Geometry check sheet. Reference: the model listing, model coordinates, mm. A direction names the side the tool comes from. Round coordinates to 2 decimals unless told otherwise and drop trailing zeros. Order: outer loops, then holes, each group sorted by start corner. A loop starts at its lowest first (then second) coordinate and runs counter-clockwise, first axis right, second up. Notation, with made-up numbers: (87, 44.5) - (101, 44.5) arc R21 cw to (101, 67.5) - close; hole circle Ø5 at (-1.75, -12). An arc over 180 degrees is marked (long way). Use a Markdown table: item, result. Add a question column.
(1) Mould release check, pull along X, two halves, no side actions. Record for faces 1 (the face through (-17.47, -40.28, 1.61)), 2 (the face through (-16, -41, 0)), 3 (the face through (-27.54, -41.19, -13.11)): released by +X, released by -X, zero draft, split by the parting line, or undercut.
(2) Gauge pin test, flat ends, axial feed: P1, Ø1.1, axis at x = -1.5, y = -30, coming from the +Z side; P2, Ø8, axis at x = -21, z = 5.5, coming from the +Y side; P3, Ø5, axis at x = -27, y = 0.5, coming from the -Z side; P4, Ø3.5, axis at x = -20, z = 0, coming from the -Y side. Record the tip position at first contact, or that the pin passes through.
(3) Section check A-A on x = -5.5. Record the boundary of the cut face in (y, z), then the cut area to 3 significant figures.
(4) Section check D-D on z = 1. Give the number of separate pieces and of enclosed holes in the cut face, then the cut area to 3 significant figures.
(5) Thickness scan on line 1 along Y through (x, z) = (-17, 2); line 2 along Y through (x, z) = (-27, 12); line 3 along Z through (x, y) = (-26.5, -30.2). Record the ranges inside material, lowest first. Write a range as [from, to].
(6) Section check B-B on z = 12.5. Record the boundary of the cut face in (x, y), then the cut area to 3 significant figures.
(7) Section check C-C on y = -12.5. Record the boundary of the cut face in (x, z).
(8) Access from +Z, -Z, +X, -X, +Y, -Y to the whole of each face (thin tool, end or side, straight path). Record for faces 4 (the face through (-8, 3, -5)), 5 (the face through (-27, -4, -13)), 6 (the face through (-19, 1, 5)).
```python
from build123d import *

# Parameters (mm, degrees)
CROQUIS1_R              = 3
CROQUIS1_R_2            = 3.1
SALIENTE_EXTRUIR1_DEPTH = 6
CROQUIS2_W              = 10
CROQUIS2_H              = 3
SALIENTE_EXTRUIR2_DEPTH = 14.2
SALIENTE_EXTRUIR3_START = 24.5
CROQUIS3_R              = 3.1
SALIENTE_EXTRUIR3_DEPTH = 24.5
CROQUIS6_R              = 8
CORTAR_EXTRUIR1_DEPTH   = 18
REDONDEO1_R             = 5
CROQUIS7_W              = 17.859034053
CROQUIS7_H              = 1
CORTAR_EXTRUIR2_DEPTH   = 1
CROQUIS8_W              = 13
CROQUIS8_H              = 6
SALIENTE_EXTRUIR4_DEPTH = 20
CROQUIS9_W              = 5
CROQUIS9_H              = 13
SALIENTE_EXTRUIR5_DEPTH = 20.2
CROQUIS10_W             = 3
CROQUIS10_H             = 14.2
CORTAR_EXTRUIR3_DEPTH   = 20
SALIENTE_EXTRUIR6_DEPTH = 5
SALIENTE_EXTRUIR7_DEPTH = 6
REDONDEO2_R             = 4
CROQUIS13_W             = 15
CROQUIS13_H             = 24.5
CORTAR_EXTRUIR4_DEPTH   = 11
REDONDEO3_R             = 4
REDONDEO4_R             = 5
REDONDEO9_SIZE          = 10
CROQUIS15_W             = 23.51054635
CROQUIS15_H             = 8.430737454
CORTAR_EXTRUIR6_DEPTH   = 12.311914061
REDONDEO10_R            = 5
CROQUIS16_W             = 33
CROQUIS16_H             = 33
SALIENTE_EXTRUIR8_DEPTH = 5
CROQUIS18_R             = 1.5
CORTAR_EXTRUIR7_DEPTH   = 10
CROQUIS19_R             = 8
CORTAR_EXTRUIR8_DEPTH   = 10
REDONDEO13_R            = 5
REDONDEO14_R            = 5
REDONDEO15_R            = 5
REDONDEO17_SIZE         = 3
CROQUIS20_W             = 26.447439695
CROQUIS20_H             = 7.153283898
CORTAR_EXTRUIR9_DEPTH   = 8
REDONDEO18_DEPTH        = 6
REDONDEO19_SIZE         = 4
REDONDEO20_SIZE         = 5
CROQUIS21_W             = 10
CROQUIS21_H             = 4.320063387
SALIENTE_EXTRUIR9_DEPTH = 9
CROQUIS14_R             = 3
CORTAR_EXTRUIR5_DEPTH   = 59


with BuildPart() as part:
    # Croquis1 → Saliente-Extruir1 (new body)
    with BuildSketch(Plane(origin=(0, 0, 0), x_dir=(1, 0, 0), z_dir=(0, 1, 0))):
        with BuildLine():
            Line((-5, 20), (-5, 0))
            ThreePointArc((-5, 0), (0, -5), (5, 0))
            Line((5, 0), (5, 20))
            ThreePointArc((5, 20), (0, 25), (-5, 20))
        make_face()
        with Locations(Location((0, 20, 0), (0, 0, 270))):
            Circle(CROQUIS1_R, mode=Mode.SUBTRACT)
        with Locations(Location((0, 0, 0), (0, 0, 270))):
            Circle(CROQUIS1_R_2, mode=Mode.SUBTRACT)
    extrude(amount=SALIENTE_EXTRUIR1_DEPTH)

    # Croquis2 → Saliente-Extruir2 (add)
    with BuildSketch(Plane.XZ):
        with Locations((0, -14.5)):
            Rectangle(CROQUIS2_W, CROQUIS2_H)
    extrude(amount=SALIENTE_EXTRUIR2_DEPTH)

    # Croquis3 → Saliente-Extruir3 (add)
    with BuildSketch(Plane.XZ.offset(14.2).offset(SALIENTE_EXTRUIR3_START)):
        with BuildLine():
            Line((-5, -5), (-5, -16))
            Line((-5, -16), (5, -16))
            Line((5, -16), (5, 0))
            ThreePointArc((5, 0), (3.535533906, 3.535533906), (0, 5))
            Line((0, 5), (-30, 5))
            Line((-30, 5), (-30, -5))
            Line((-30, -5), (-5, -5))
        make_face()
        with Locations(Location((0, 0, 0), (0, 0, 90))):
            Circle(CROQUIS3_R, mode=Mode.SUBTRACT)
    extrude(amount=-SALIENTE_EXTRUIR3_DEPTH)

    # Croquis6 → Cortar-Extruir1 (cut)
    with BuildSketch(Plane.XY.offset(5)):
        with Locations((-20, -30.2)):
            Circle(CROQUIS6_R)
    extrude(amount=-CORTAR_EXTRUIR1_DEPTH, mode=Mode.SUBTRACT)

    # Redondeo1
    redondeo1_edges = [part.edges().sort_by_distance(p)[0] for p in [
        (-5, -26.45, -5),
    ]]
    fillet(redondeo1_edges, radius=REDONDEO1_R)

    # Croquis7 → Cortar-Extruir2 (cut)
    with BuildSketch(Plane.XY.offset(5)):
        with Locations((-3.905990917, -30.2)):
            Rectangle(CROQUIS7_W, CROQUIS7_H)
    extrude(amount=-CORTAR_EXTRUIR2_DEPTH, mode=Mode.SUBTRACT)

    # Croquis8 → Saliente-Extruir4 (add)
    with BuildSketch(Plane.ZY.offset(5)):
        with Locations((-6.5, 3)):
            Rectangle(CROQUIS8_W, CROQUIS8_H)
    extrude(amount=SALIENTE_EXTRUIR4_DEPTH)

    # Croquis9 → Saliente-Extruir5 (add)
    with BuildSketch(Plane(origin=(0, 6, 0), x_dir=(1, 0, 0), z_dir=(0, 1, 0))):
        with Locations((-27.5, 6.5)):
            Rectangle(CROQUIS9_W, CROQUIS9_H)
    extrude(amount=-SALIENTE_EXTRUIR5_DEPTH)

    # Croquis10 → Cortar-Extruir3 (cut)
    with BuildSketch(Plane.ZY.offset(5)):
        with Locations((-14.5, -7.1)):
            Rectangle(CROQUIS10_W, CROQUIS10_H)
    extrude(amount=-CORTAR_EXTRUIR3_DEPTH, mode=Mode.SUBTRACT)

    # Croquis11 → Saliente-Extruir6 (add)
    with BuildSketch(Plane.XY):
        Polygon((-5, 0), (-5, 6), (-30, 6), (-30, -14.2), (-25, -14.2), (-25, 0), align=None)
    extrude(amount=SALIENTE_EXTRUIR6_DEPTH)

    # Croquis12 → Saliente-Extruir7 (add)
    with BuildSketch(Plane(origin=(0, 6, 0), x_dir=(1, 0, 0), z_dir=(0, 1, 0))):
        Polygon((-5, -5), (0, -5), (-4.695965468, 0.35178881), (-6.407055534, -0.228241721), align=None)
    extrude(amount=-SALIENTE_EXTRUIR7_DEPTH)

    # Redondeo2
    # the kernel refuses this fillet: 4 mm, written as the material it adds along each edge
    with BuildSketch(Plane(origin=(-30, -14.2, -5), x_dir=(0, 0, -1), z_dir=(1, 0, 0))) as redondeo2_piece_1:
        with BuildLine():
            CenterArc((REDONDEO2_R, -REDONDEO2_R), REDONDEO2_R, 90, 90)
            Line((0, -REDONDEO2_R), (0, 0))
            Line((0, 0), (REDONDEO2_R, 0))
        make_face()
    extrude(amount=5)

    # Croquis13 → Cortar-Extruir4 (cut)
    with BuildSketch(Plane(origin=(0, 0, -16), x_dir=(-1, 0, 0), z_dir=(0, 0, -1))):
        with Locations((2.5, -26.45)):
            Rectangle(CROQUIS13_W, CROQUIS13_H)
    extrude(amount=-CORTAR_EXTRUIR4_DEPTH, mode=Mode.SUBTRACT)

    # Redondeo3
    redondeo3_edges = [part.edges().sort_by_distance(p)[0] for p in [
        (-5, 3, -13),
    ]]
    fillet(redondeo3_edges, radius=REDONDEO3_R)

    # Redondeo4
    redondeo4_edges = [part.edges().sort_by_distance(p)[0] for p in [
        (5, -26.45, -5),
    ]]
    fillet(redondeo4_edges, radius=REDONDEO4_R - 0.0001)  # a hair under: the kernel refuses the full size

    # Redondeo9
    # a fillet whose section is not a circle: 10 mm, written as the material it takes off along each edge
    with BuildSketch(Plane(origin=(-30, 6, 30), x_dir=(0, -1, 0), z_dir=(0, 0, -1))) as redondeo9_piece_1:
        with BuildLine():
            Bezier((REDONDEO9_SIZE, 0), (0, 0), (0, -REDONDEO9_SIZE), weights=[1, 1, 1])
            Line((0, -REDONDEO9_SIZE), (0, 0))
            Line((0, 0), (REDONDEO9_SIZE, 0))
        make_face()
    extrude(amount=68, mode=Mode.SUBTRACT)

    # Croquis15 → Cortar-Extruir6 (cut)
    with BuildSketch(Plane.XY.offset(-25.311914061)):
        with Locations((-4.843890072, 4.215368727)):
            Rectangle(CROQUIS15_W, CROQUIS15_H)
    extrude(amount=CORTAR_EXTRUIR6_DEPTH, mode=Mode.SUBTRACT)

    # Redondeo10
    redondeo10_edges = [part.edges().sort_by_distance(p)[0] for p in [
        (5, 3, -13),
    ]]
    fillet(redondeo10_edges, radius=REDONDEO10_R)

    # Croquis16 → Saliente-Extruir8 (add)
    with BuildSketch(Plane.ZY.offset(30)):
        with Locations((0, -30.2)):
            Rectangle(CROQUIS16_W, CROQUIS16_H)
    extrude(amount=-SALIENTE_EXTRUIR8_DEPTH)

    # Croquis18 → Cortar-Extruir7 (cut)
    with BuildSketch(Plane.ZY.offset(30)):
        with Locations((12, -42.2)):
            Circle(CROQUIS18_R)
        with Locations((-12, -42.2)):
            Circle(CROQUIS18_R)
        with Locations((-12, -18.2)):
            Circle(CROQUIS18_R)
        with Locations((12, -18.2)):
            Circle(CROQUIS18_R)
    extrude(amount=-CORTAR_EXTRUIR7_DEPTH, mode=Mode.SUBTRACT)

    # Croquis19 → Cortar-Extruir8 (cut)
    with BuildSketch(Plane.ZY.offset(30)):
        with Locations((0, -30.2)):
            Circle(CROQUIS19_R)
    extrude(amount=-CORTAR_EXTRUIR8_DEPTH, mode=Mode.SUBTRACT)

    # Redondeo13
    redondeo13_edges = [part.edges().sort_by_distance(p)[0] for p in [
        (-27.5, -13.7, 16.5),
    ]]
    fillet(redondeo13_edges, radius=REDONDEO13_R)

    # Redondeo14
    redondeo14_edges = [part.edges().sort_by_distance(p)[0] for p in [
        (-27.5, -46.7, 16.5),
    ]]
    fillet(redondeo14_edges, radius=REDONDEO14_R)

    # Redondeo15
    redondeo15_edges = [part.edges().sort_by_distance(p)[0] for p in [
        (-27.5, -46.7, -16.5),
    ]]
    fillet(redondeo15_edges, radius=REDONDEO15_R)

    # Redondeo17
    # a fillet whose section is not a circle: 3 mm, written as the material it takes off along each edge
    with BuildSketch(Plane(origin=(-37.5, -13.7, -16.5), x_dir=(0, -1, 0), z_dir=(1, 0, 0))) as redondeo17_piece_1:
        with BuildLine():
            Bezier((REDONDEO17_SIZE, 0), (0, 0), (0, -REDONDEO17_SIZE), weights=[1, 1, 1])
            Line((0, -REDONDEO17_SIZE), (0, 0))
            Line((0, 0), (REDONDEO17_SIZE, 0))
        make_face()
    extrude(amount=20, mode=Mode.SUBTRACT)

    # Croquis20 → Cortar-Extruir9 (cut)
    with BuildSketch(Plane(origin=(0, 0, -13), x_dir=(-1, 0, 0), z_dir=(0, 0, -1))):
        with Locations((6.776280153, 2.423358051)):
            Rectangle(CROQUIS20_W, CROQUIS20_H)
    extrude(amount=-CORTAR_EXTRUIR9_DEPTH, mode=Mode.SUBTRACT)

    # Redondeo18: read off the stored shape, not the designer's step
    # Redondeo18 outline → Redondeo18 (add)
    with BuildSketch(Plane(origin=(0, 0, 0), x_dir=(1, 0, 0), z_dir=(0, 1, 0))):
        with BuildLine():
            Line((-20, 5), (-16, 5))
            add(Edge.make_bspline(
                [(-16, 5), (-20, 5), (-20, 9)],
                knots=[0, 0, 0, 1, 1, 1], degree=2))
            Line((-20, 9), (-20, 5))
        make_face()
    extrude(amount=REDONDEO18_DEPTH)

    # Redondeo19
    # a fillet whose section is not a circle: 4 mm, written as the material it takes off along each edge
    with BuildSketch(Plane(origin=(-20, -10, -13), x_dir=(0, 0, 1), z_dir=(0, 1, 0))) as redondeo19_piece_1:
        with BuildLine():
            Bezier((REDONDEO19_SIZE, 0), (0, 0), (0, -REDONDEO19_SIZE), weights=[1, 1, 1])
            Line((0, -REDONDEO19_SIZE), (0, 0))
            Line((0, 0), (REDONDEO19_SIZE, 0))
        make_face()
    extrude(amount=26, mode=Mode.SUBTRACT)

    # Redondeo20
    # a fillet whose section is not a circle: 5 mm, written as the material it takes off along each edge
    with BuildSketch(Plane(origin=(5, 18.5, -5), x_dir=(-1, 0, 0), z_dir=(0, -1, 0))) as redondeo20_piece_1:
        with BuildLine():
            Bezier((REDONDEO20_SIZE, 0), (0, 0), (0, -REDONDEO20_SIZE), weights=[1, 1, 1])
            Line((0, -REDONDEO20_SIZE), (0, 0))
            Line((0, 0), (REDONDEO20_SIZE, 0))
        make_face()
    extrude(amount=31, mode=Mode.SUBTRACT)

    # Croquis21 → Saliente-Extruir9 (add)
    with BuildSketch(Plane(origin=(-25, 0, 0), x_dir=(0, 0, -1), z_dir=(1, 0, 0))):
        with Locations((0, -40.860031694)):
            Rectangle(CROQUIS21_W, CROQUIS21_H)
    extrude(amount=SALIENTE_EXTRUIR9_DEPTH)

    # Croquis14 → Cortar-Extruir5 (cut)
    with BuildSketch(Plane(origin=(0, 6, 0), x_dir=(1, 0, 0), z_dir=(0, 1, 0))):
        with Locations(Location((-20, 0, 0), (0, 0, 270))):
            Circle(CROQUIS14_R)
    extrude(amount=-CORTAR_EXTRUIR5_DEPTH, mode=Mode.SUBTRACT)


solid = part.part
```
Check sheet entries:
| question | item | result |
|---|---|---|
| 1 | face 1 | undercut |
| 1 | face 2 | released by +X |
| 1 | face 3 | zero draft |
| 2 | P1 | stops at z = 5 |
| 2 | P2 | stops at y = 6 |
| 2 | P3 | stops at z = -13 |
| 2 | P4 | passes through |
| 3 | outline | (-38.7, -5) - (-14.2, -5) - (-14.2, 5) - (-29.7, 5) - (-29.7, 4) - (-30.7, 4) - (-30.7, 5) - (-38.7, 5) - close; (0, -5) - (6, -5) - (6, 5) - (0, 5) - close |
| 3 | area | 304 mm2 |
| 4 | separate pieces | 6 |
| 4 | enclosed holes | 0 |
| 4 | area | 652 mm2 |
| 5 | line 1 | y = [-43.02, -37.62], [-22.78, -14.2], [0, 6] |
| 5 | line 2 | y = [-46.67, -43.7], [-40.7, -19.7], [-16.7, -13.73] |
| 5 | line 3 | z = [-16.5, -8], [8, 16.5] |
| 6 | outline | (-30, -46.6) - (-25, -46.6) - (-25, -43.61) - (-30, -43.61) - close; (-30, -40.79) - (-25, -40.79) - (-25, -19.61) - (-30, -19.61) - close; (-30, -16.79) - (-25, -16.79) - (-25, -13.8) - (-30, -13.8) - close |
| 6 | area | 136 mm2 |
| 7 | outline | (-30, -13) - (-25, -13) - (-25, 5) - (-30, 5) - close |
| 8 | face 4 | -Z, +X, +Y, -Y |
| 8 | face 5 | -Z, +X, -X, +Y |
| 8 | face 6 | +Z, +X, -X, +Y |
